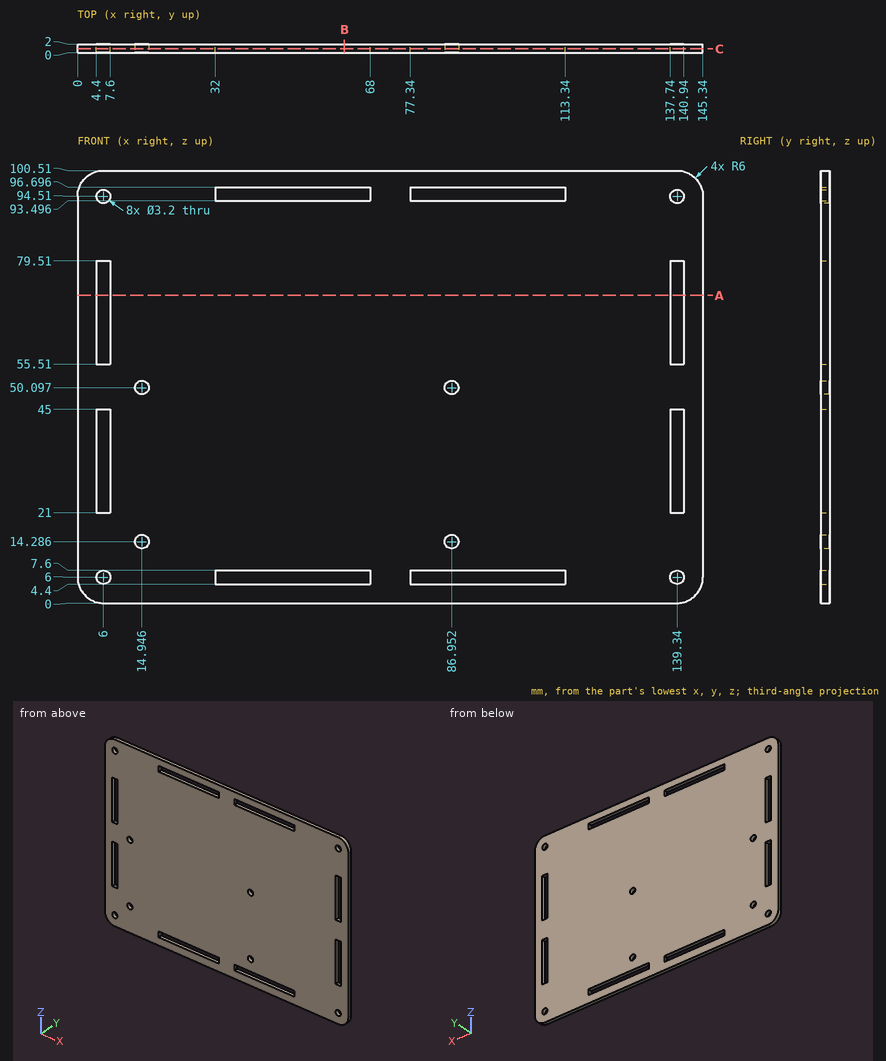
Answer from the drawing. Dimensions are ordinates in mm from the lowest x, y and z of the part. Round coordinates to 2 decimals unless told otherwise and drop trailing zeros. Write each loop counter-clockwise with the first axis right and the second up, starting at its lowest first coordinate (ties: lowest second). Pieces come first, ordered by that corner, then holes. Notation, with made-up numbers: (85, 81.25) - (113, 81.25) arc R22 ccw to (113, 90.25) - close; hole circle Ø7 at (66, -11). An arc over 180 degrees is marked (long way). Use a Markdown table: item, result.
(1) The part is cut by section C-C (y = 0.85). State how many separate pieces and enclosed holes the cut face has, then the cut area to 3 significant figures.
Reported:
| item | result |
|---|---|
| separate pieces | 1 |
| enclosed holes | 16 |
| area | 13,700 mm2 |
(2) The part is cut by section B-B (x = 62). Write down the section's boundary in (y, z).
Reported:
| item | result |
|---|---|
| outline | (0, 0) - (2, 0) - (2, 4.4) - (0, 4.4) - close; (0, 7.6) - (2, 7.6) - (2, 93.5) - (0, 93.5) - close; (0, 96.7) - (2, 96.7) - (2, 100.51) - (0, 100.51) - close |
(3) The part is cut by section A-A (z = 71.5). Write down the section's boundary in (x, y), then the cut area to 3 significant figures.
Reported:
| item | result |
|---|---|
| outline | (0, 0) - (4.4, 0) - (4.4, 2) - (0, 2) - close; (7.6, 0) - (137.74, 0) - (137.74, 2) - (7.6, 2) - close; (140.94, 0) - (145.34, 0) - (145.34, 2) - (140.94, 2) - close |
| area | 278 mm2 |
(4) This flat-tipped pin is pushed along its axis until it touches: pin 1 Ø1 at (y, z) = (1, 95.5) entering from -X. Where does it stop, or does it pass through?
Reported:
| item | result |
|---|---|
| pin 1 | x = 0.02 |
(5) Straight lines are drawn through the part: line 1 along X through (y, z) = (1.55, 23); line 2 along X through (y, z) = (0.75, 6); line 3 along X through (y, z) = (1, 50) (3 decimals). For each, find the intervals that lie inside material, in ascending order. Write a range as [from, to].
Reported:
| item | result |
|---|---|
| line 1 | [0, 4.4], [7.6, 137.74], [140.94, 145.34] |
| line 2 | [0, 4.4], [7.6, 32], [68, 77.34], [113.34, 137.74], [140.94, 145.34] |
| line 3 | [0, 13.349], [16.543, 85.355], [88.549, 145.34] |
